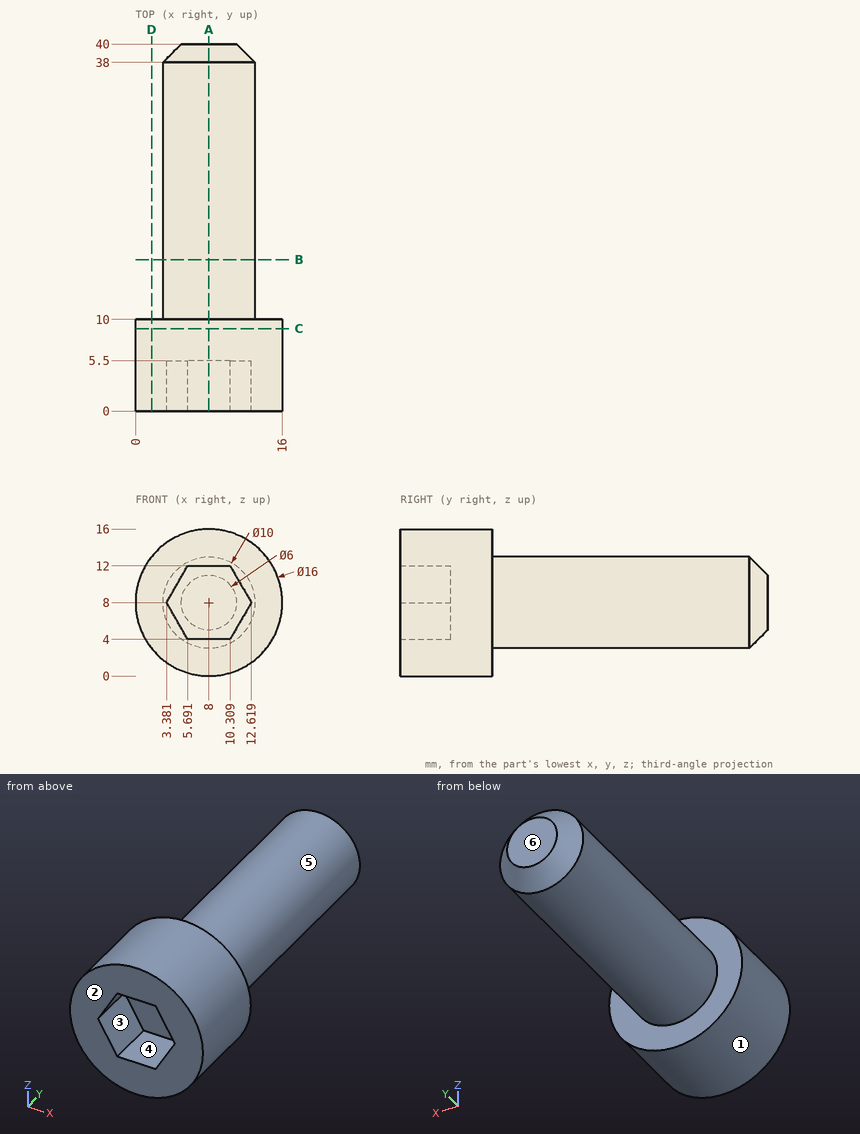
Drawing for the job (mm, zero at the part's lowest x, y, z). A direction names the side the tool comes from. Give positions to 0.01 mm unless a question says otherwise; leave off trailing zeros. Order: outer loops, then holes, each group sorted by start corner. A loop starts at its lowest first (then second) coordinate and runs counter-clockwise, first axis right, second up. Notation, with made-up numbers: M 38.25,43.25 L 93.25,43.25 A27 cw 93.25,67.25 Z; hole C -15.75,14.25 d11. An arc over 180 degrees is marked long. Write item = value, one per line. Start each with the question number.
(1) Probe L1, parallel to Y at x = 9.75, z = 6.25; L2, parallel to Z at x = 12, y = 13.5; L3, parallel to Y at x = 4.5, z = 12. List the from-to ranges inside material, lowest first. Write a range as [from, to].
(2) Slice it at D-D on x = 1.75. Write the cut outline in (y, z).
(3) Which spindle directions (+Z, -Z, +X, -X, +Y, -Y) get a long thin tool onto all of the face, cutting with end or side? Do the marked faces 4, 5 and 6. Say none if no direction does.
(4) Slice it at C-C on y = 9. Write the cut outline in (x, z).
(5) Two-plate mould, pull along Z, no slides. Class the marked faces 1, 2 and 3: released by +Z, released by -Z, zero draft, split by the parting line, or undercut.
(6) Pin check, flat tips, straight feed: pin 1 Ø3 at (x, z) = (13.5, 13) entering from +Y; pin 2 Ø1.5 at (y, z) = (27, 9.5) entering from +X; pin 3 Ø6 at (x, y) = (2.5, 20.5) entering from -Z. Stop position of each tip, or through.
(7) Slice it at B-B on y = 16.5. Write the cut outline in (x, z).
(8) Slice it at A-A on x = 8. Write the cut outline in (y, z), plus the area to 3 significant figures.
Responses:
q1.L1 = [5.5, 40]
q1.L2 = [5, 11]
q1.L3 = [0, 10]
q2.outline = M 0,3.01 L 10,3.01 L 10,12.99 L 0,12.99 Z
q3.face_4 = -Y
q3.face_5 = +Y
q3.face_6 = +Z, -Z, +X, -X, +Y
q4.outline = C 8,8 d16
q5.face_1 = split by the parting line
q5.face_2 = zero draft
q5.face_3 = undercut
q6.pin_1 = 10
q6.pin_2 = 12.94
q6.pin_3 = 3.67
q7.outline = C 8,8 d10
q8.outline = M 0,0 L 10,0 L 10,3 L 38,3 L 40,5 L 40,11 L 38,13 L 10,13 L 10,16 L 0,16 L 0,12 L 5.5,12 L 5.5,4 L 0,4 Z
q8.area = 412 mm2
